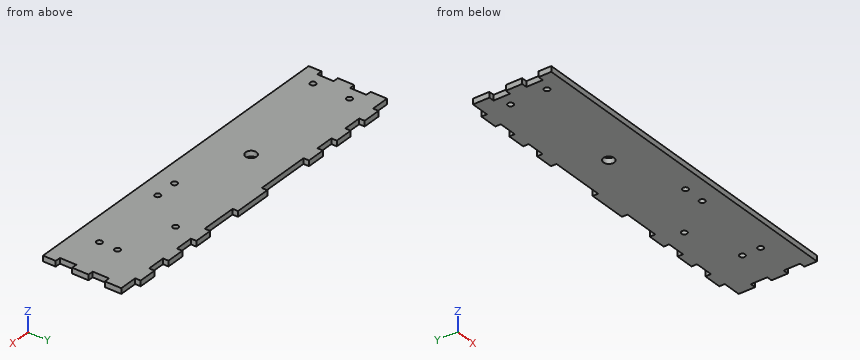
from build123d import *

# Parameters (mm, degrees)
SKETCH1_W           = 191
SKETCH1_H           = 46
SKETCH1_R           = 1.549999948
BOSS_EXTRUDE1_DEPTH = 3
CUT_EXTRUDE1_REACH  = 5
SKETCH3_W           = 10
SKETCH3_H           = 3
SKETCH3_W_2         = 30
SKETCH3_W_3         = 20
SKETCH4_W           = 3
SKETCH4_H           = 9
CUT_EXTRUDE2_DEPTH  = 3
CUT_EXTRUDE3_REACH  = 5
SKETCH6_R           = 3
CUT_EXTRUDE4_REACH  = 5
SKETCH7_R           = 1.55


with BuildPart() as part:
    # Sketch1 → Boss-Extrude1 (new body)
    with BuildSketch(Plane.XY):
        with Locations((-95.5, 23)):
            Rectangle(SKETCH1_W, SKETCH1_H)
        with Locations((-181, 30)):
            Circle(SKETCH1_R, mode=Mode.SUBTRACT)
        with Locations((-181, 10)):
            Circle(SKETCH1_R, mode=Mode.SUBTRACT)
    extrude(amount=BOSS_EXTRUDE1_DEPTH)

    # Sketch3 → Cut-Extrude1 (cut, up to next)
    with BuildSketch(Plane(origin=(0, 0, 0), x_dir=(-1, 0, 0), z_dir=(0, 0, -1)), mode=Mode.PRIVATE) as cut_extrude1_sk1:
        with Locations((45, 44.5)):
            Rectangle(SKETCH3_W, SKETCH3_H)
    cut_extrude1_tool1 = extrude(cut_extrude1_sk1.sketch, amount=-CUT_EXTRUDE1_REACH, mode=Mode.PRIVATE) & part.part
    add(cut_extrude1_tool1.solids().sort_by_distance((-45, 44.5, 0))[0], mode=Mode.SUBTRACT)
    # Sketch3 → Cut-Extrude1 (cut, up to next)
    with BuildSketch(Plane(origin=(0, 0, 0), x_dir=(-1, 0, 0), z_dir=(0, 0, -1)), mode=Mode.PRIVATE) as cut_extrude1_sk2:
        with Locations((25, 44.5)):
            Rectangle(SKETCH3_W, SKETCH3_H)
    cut_extrude1_tool2 = extrude(cut_extrude1_sk2.sketch, amount=-CUT_EXTRUDE1_REACH, mode=Mode.PRIVATE) & part.part
    add(cut_extrude1_tool2.solids().sort_by_distance((-25, 44.5, 0))[0], mode=Mode.SUBTRACT)
    # Sketch3 → Cut-Extrude1 (cut, up to next)
    with BuildSketch(Plane(origin=(0, 0, 0), x_dir=(-1, 0, 0), z_dir=(0, 0, -1)), mode=Mode.PRIVATE) as cut_extrude1_sk3:
        with Locations((5, 44.5)):
            Rectangle(SKETCH3_W, SKETCH3_H)
    cut_extrude1_tool3 = extrude(cut_extrude1_sk3.sketch, amount=-CUT_EXTRUDE1_REACH, mode=Mode.PRIVATE) & part.part
    add(cut_extrude1_tool3.solids().sort_by_distance((-5, 44.5, 0))[0], mode=Mode.SUBTRACT)
    # Sketch3 → Cut-Extrude1 (cut, up to next)
    with BuildSketch(Plane(origin=(0, 0, 0), x_dir=(-1, 0, 0), z_dir=(0, 0, -1)), mode=Mode.PRIVATE) as cut_extrude1_sk4:
        with Locations((166, 44.5)):
            Rectangle(SKETCH3_W, SKETCH3_H)
    cut_extrude1_tool4 = extrude(cut_extrude1_sk4.sketch, amount=-CUT_EXTRUDE1_REACH, mode=Mode.PRIVATE) & part.part
    add(cut_extrude1_tool4.solids().sort_by_distance((-166, 44.5, 0))[0], mode=Mode.SUBTRACT)
    # Sketch3 → Cut-Extrude1 (cut, up to next)
    with BuildSketch(Plane(origin=(0, 0, 0), x_dir=(-1, 0, 0), z_dir=(0, 0, -1)), mode=Mode.PRIVATE) as cut_extrude1_sk5:
        with Locations((146, 44.5)):
            Rectangle(SKETCH3_W, SKETCH3_H)
    cut_extrude1_tool5 = extrude(cut_extrude1_sk5.sketch, amount=-CUT_EXTRUDE1_REACH, mode=Mode.PRIVATE) & part.part
    add(cut_extrude1_tool5.solids().sort_by_distance((-146, 44.5, 0))[0], mode=Mode.SUBTRACT)
    # Sketch3 → Cut-Extrude1 (cut, up to next)
    with BuildSketch(Plane(origin=(0, 0, 0), x_dir=(-1, 0, 0), z_dir=(0, 0, -1)), mode=Mode.PRIVATE) as cut_extrude1_sk6:
        with Locations((116, 44.5)):
            Rectangle(SKETCH3_W_2, SKETCH3_H)
    cut_extrude1_tool6 = extrude(cut_extrude1_sk6.sketch, amount=-CUT_EXTRUDE1_REACH, mode=Mode.PRIVATE) & part.part
    add(cut_extrude1_tool6.solids().sort_by_distance((-116, 44.5, 0))[0], mode=Mode.SUBTRACT)
    # Sketch3 → Cut-Extrude1 (cut, up to next)
    with BuildSketch(Plane(origin=(0, 0, 0), x_dir=(-1, 0, 0), z_dir=(0, 0, -1)), mode=Mode.PRIVATE) as cut_extrude1_sk7:
        with Locations((70, 44.5)):
            Rectangle(SKETCH3_W_3, SKETCH3_H)
    cut_extrude1_tool7 = extrude(cut_extrude1_sk7.sketch, amount=-CUT_EXTRUDE1_REACH, mode=Mode.PRIVATE) & part.part
    add(cut_extrude1_tool7.solids().sort_by_distance((-70, 44.5, 0))[0], mode=Mode.SUBTRACT)
    # Sketch3 → Cut-Extrude1 (cut, up to next)
    with BuildSketch(Plane(origin=(0, 0, 0), x_dir=(-1, 0, 0), z_dir=(0, 0, -1)), mode=Mode.PRIVATE) as cut_extrude1_sk8:
        with Locations((186, 44.5)):
            Rectangle(SKETCH3_W, SKETCH3_H)
    cut_extrude1_tool8 = extrude(cut_extrude1_sk8.sketch, amount=-CUT_EXTRUDE1_REACH, mode=Mode.PRIVATE) & part.part
    add(cut_extrude1_tool8.solids().sort_by_distance((-186, 44.5, 0))[0], mode=Mode.SUBTRACT)

    # Sketch4 → Cut-Extrude2 (cut)
    with BuildSketch(Plane.XY.offset(3)):
        with Locations((-1.5, 29.5)):
            Rectangle(SKETCH4_W, SKETCH4_H)
        with Locations((-1.5, 11.5)):
            Rectangle(SKETCH4_W, SKETCH4_H)
    cut_extrude2 = extrude(amount=-CUT_EXTRUDE2_DEPTH, mode=Mode.SUBTRACT)

    # Mirror1: Cut-Extrude2 across plane
    add(cut_extrude2.mirror(Plane(origin=(-95.5, 0, 0), x_dir=(0, 0, 1), z_dir=(1, 0, 0))), mode=Mode.SUBTRACT)

    # Sketch6 → Cut-Extrude3 (cut, up to next)
    with BuildSketch(Plane.XY.offset(3), mode=Mode.PRIVATE) as cut_extrude3_sk1:
        with Locations((-119.5, 23)):
            Circle(SKETCH6_R)
    cut_extrude3_tool1 = extrude(cut_extrude3_sk1.sketch, amount=-CUT_EXTRUDE3_REACH, mode=Mode.PRIVATE) & part.part
    add(cut_extrude3_tool1.solids().sort_by_distance((-119.5, 23, 3))[0], mode=Mode.SUBTRACT)

    # Sketch7 → Cut-Extrude4 (cut, up to next)
    with BuildSketch(Plane.XY.offset(3), mode=Mode.PRIVATE) as cut_extrude4_sk1:
        with Locations((-53.5, 32)):
            Circle(SKETCH7_R)
    cut_extrude4_tool1 = extrude(cut_extrude4_sk1.sketch, amount=-CUT_EXTRUDE4_REACH, mode=Mode.PRIVATE) & part.part
    add(cut_extrude4_tool1.solids().sort_by_distance((-53.5, 32, 3))[0], mode=Mode.SUBTRACT)
    # Sketch7 → Cut-Extrude4 (cut, up to next)
    with BuildSketch(Plane.XY.offset(3), mode=Mode.PRIVATE) as cut_extrude4_sk2:
        with Locations((-68.757359313, 10.5)):
            Circle(SKETCH7_R)
    cut_extrude4_tool2 = extrude(cut_extrude4_sk2.sketch, amount=-CUT_EXTRUDE4_REACH, mode=Mode.PRIVATE) & part.part
    add(cut_extrude4_tool2.solids().sort_by_distance((-68.757359, 10.5, 3))[0], mode=Mode.SUBTRACT)
    # Sketch7 → Cut-Extrude4 (cut, up to next)
    with BuildSketch(Plane.XY.offset(3), mode=Mode.PRIVATE) as cut_extrude4_sk3:
        with Locations((-80.757359313, 10.5)):
            Circle(SKETCH7_R)
    cut_extrude4_tool3 = extrude(cut_extrude4_sk3.sketch, amount=-CUT_EXTRUDE4_REACH, mode=Mode.PRIVATE) & part.part
    add(cut_extrude4_tool3.solids().sort_by_distance((-80.757359, 10.5, 3))[0], mode=Mode.SUBTRACT)
    # Sketch7 → Cut-Extrude4 (cut, up to next)
    with BuildSketch(Plane.XY.offset(3), mode=Mode.PRIVATE) as cut_extrude4_sk4:
        with Locations((-23.5, 23)):
            Circle(SKETCH7_R)
    cut_extrude4_tool4 = extrude(cut_extrude4_sk4.sketch, amount=-CUT_EXTRUDE4_REACH, mode=Mode.PRIVATE) & part.part
    add(cut_extrude4_tool4.solids().sort_by_distance((-23.5, 23, 3))[0], mode=Mode.SUBTRACT)
    # Sketch7 → Cut-Extrude4 (cut, up to next)
    with BuildSketch(Plane.XY.offset(3), mode=Mode.PRIVATE) as cut_extrude4_sk5:
        with Locations((-23.5, 13)):
            Circle(SKETCH7_R)
    cut_extrude4_tool5 = extrude(cut_extrude4_sk5.sketch, amount=-CUT_EXTRUDE4_REACH, mode=Mode.PRIVATE) & part.part
    add(cut_extrude4_tool5.solids().sort_by_distance((-23.5, 13, 3))[0], mode=Mode.SUBTRACT)


solid = part.part
Read the model definition and answer for the solid it produces. Units are mm, in the model's axes. Coordinates: 2 decimals unless noted, no trailing zeros. Loops run counter-clockwise (first coordinate to the right, second up) from the corner with the lowest first, then second, coordinate; pieces in that order, holes last.
Q1. Each of these flat-tipped pins is pushed along its axis until it touches: pin 1 Ø1.5 at (y, z) = (31, 1) entering from -X; pin 2 Ø0.9 at (y, z) = (13.5, 2) entering from +X; pin 3 Ø1.5 at (y, z) = (44.5, 1.5) entering from +X. Where does it stop, or does it pass through?
Q2. Consider probe 1 along Y at (x, z) = (-119.5, 1.4); probe 2 along X at (y, z) = (23.5, 1.3); probe 3 along Y at (x, z) = (-116, 2.2). Determine where each line is inside the solid, lowest interval first.
Q3. The part is cut by section B-B on z = 2.5. Give the number of separate pieces and of enclosed holes in the cut face, and give its area (3 significant figures).
Q4. The part is cut by section C-C on x = -44. Write down the section's boundary in (y, z).
Q5. The part is cut by section A-A on x = -119.5. Write down the section's boundary in (y, z), and give its area (3 significant figures).
Results below:
1. pin 1: stops at x = -188
1. pin 2: stops at x = -3
1. pin 3: stops at x = -10
2. probe 1: y = 0 to 20, 26 to 43
2. probe 2: x = -191 to -122.46, -116.54 to -24.97, -22.03 to 0
2. probe 3: y = 0 to 43
3. separate pieces: 1
3. enclosed holes: 8
3. area: 8,270 mm2
4. outline: (0, 0) - (43, 0) - (43, 3) - (0, 3) - close
5. outline: (0, 0) - (20, 0) - (20, 3) - (0, 3) - close; (26, 0) - (43, 0) - (43, 3) - (26, 3) - close
5. area: 111 mm2
